```python
from build123d import *

# Parameters (mm, degrees)
PAD_DEPTH    = 5
SKETCH001_R  = 1.7
HOLE_DEPTH   = 72.8243
SKETCH002_W  = 30
SKETCH002_H  = 5
PAD001_DEPTH = 5
SKETCH003_W  = 5
SKETCH003_H  = 30
PAD002_DEPTH = 30


with BuildPart() as part:
    # Sketch → Pad (new body)
    with BuildSketch(Plane.XY):
        with BuildLine():
            Line((-15, 0), (0, 0))
            Line((0, 0), (0, 15))
            Line((0, 15), (-10, 15))
            ThreePointArc((-10, 15), (-13.535534, 13.535534), (-15, 10))
            Line((-15, 10), (-15, 0))
        make_face()
    pad = extrude(amount=PAD_DEPTH)

    # Mirrored: Pad across XZ
    add(pad.mirror(Plane.XZ))

    # Sketch001 (on Face5 of Mirrored) → Hole (cut, through all)
    with BuildSketch(Plane.XY.offset(5)):
        with Locations((-7.5, 7.5)):
            Circle(SKETCH001_R)
    hole = extrude(amount=-HOLE_DEPTH, mode=Mode.SUBTRACT)

    # Mirrored001: Hole across XZ
    add(hole.mirror(Plane.XZ), mode=Mode.SUBTRACT)

    # Sketch002 (on Face2 of Mirrored001) → Pad001 (join)
    with BuildSketch(Plane.YZ):
        with Locations((0, 2.5)):
            Rectangle(SKETCH002_W, SKETCH002_H)
    extrude(amount=PAD001_DEPTH)

    # Sketch003 (on Face12 of Pad001) → Pad002 (join)
    with BuildSketch(Plane.XY.offset(5)):
        with Locations((2.5, 0)):
            Rectangle(SKETCH003_W, SKETCH003_H)
    extrude(amount=PAD002_DEPTH)


solid = part.part
```
Verification items for the finished model (mm, model axes). A direction names the side the tool comes from. Give positions to 0.01 mm unless a question says otherwise; leave off trailing zeros. Order: outer loops, then holes, each group sorted by start corner. A loop starts at its lowest first (then second) coordinate and runs counter-clockwise, first axis right, second up. Notation, with made-up numbers: M 31,14.5 L 59,14.5 A30 cw 59,49.5 Z; hole C 1,89.5 d6. An arc over 180 degrees is marked long. Answer in a Markdown table with one row per item. Add a question column.
Item 1: Mould release check, pull along X, two halves, no side actions. Record for faces 3 (the flat face through (1, 15, 13)), 4 (the cylindrical face through (-13, -14, 2)), 5 (the flat face through (5, 0, 17)), 6 (the cylindrical face through (-7.87, -5.84, 2.54)): released by +X, released by -X, zero draft, split by the parting line, or undercut.
Item 2: Scan lines: probe 1 along Y at (x, z) = (-7.5, 3.4); probe 2 along X at (y, z) = (-7.5, 1.85); probe 3 along Z at (x, y) = (-1.5, 7). Record each from-to range of solid material in increasing order. Write a range as from..to.
Item 3: Gauge pin test, flat ends, axial feed: pin 1 (2 mm diameter, centred on x = -7.5, y = -7.5, fed in from -Z); pin 2 (12 mm diameter, centred on x = -6.5, y = -5.5, fed in from +Z); pin 3 (4 mm diameter, centred on y = 3.5, z = 16.5, fed in from -X); pin 4 (10 mm diameter, centred on x = -4, z = 21.5, fed in from -Y). Record the tip position at first contact, or that the pin passes through.
Item 4: Section check B-B, the plane y = 7.5. Enter the section's corners in (x, z), and give its area (3 significant figures).
Item 5: Tool access check on faces 1 (the flat face through (-15, 0, 2)), 2 (the flat face through (-8, 0, 5)). Record the directions out of +Z, -Z, +X, -X, +Y, -Y that give a thin tool (end or side, any length) a straight path to the whole face; none if there is none.
Item 6: Section check D-D, the plane y = 0. Enter the section's corners in (x, z).
Item 7: Section check C-C, the plane z = 4. Enter the section's corners in (x, y).
Item 8: Section check A-A, the plane x = -7.5. Enter the section's corners in (y, z), and give its area (3 significant figures).
Filled sheet:
| question | item | result |
|---|---|---|
| 1 | face 3 | zero draft |
| 1 | face 4 | released by -X |
| 1 | face 5 | released by +X |
| 1 | face 6 | undercut |
| 2 | probe 1 | y = -15..-9.2, -5.8..5.8, 9.2..15 |
| 2 | probe 2 | x = -15..-9.2, -5.8..5 |
| 2 | probe 3 | z = 0..5 |
| 3 | pin 1 | passes through |
| 3 | pin 2 | stops at z = 5 |
| 3 | pin 3 | stops at x = 0 |
| 3 | pin 4 | stops at y = -15 |
| 4 | outline | M -15,0 L -9.2,0 L -9.2,5 L -15,5 Z; M -5.8,0 L 5,0 L 5,35 L 0,35 L 0,5 L -5.8,5 Z |
| 4 | area | 233 mm^2 |
| 5 | face 1 | +Z, -Z, -X, +Y, -Y |
| 5 | face 2 | +Z, -X, +Y, -Y |
| 6 | outline | M -15,0 L 5,0 L 5,35 L 0,35 L 0,5 L -15,5 Z |
| 7 | outline | M -15,-10 A5 ccw -10,-15 L 5,-15 L 5,15 L -10,15 A5 ccw -15,10 Z; hole C -7.5,-7.5 d3.4; hole C -7.5,7.5 d3.4 |
| 8 | outline | M -15,0 L -9.2,0 L -9.2,5 L -15,5 Z; M -5.8,0 L 5.8,0 L 5.8,5 L -5.8,5 Z; M 9.2,0 L 15,0 L 15,5 L 9.2,5 Z |
| 8 | area | 116 mm^2 |
